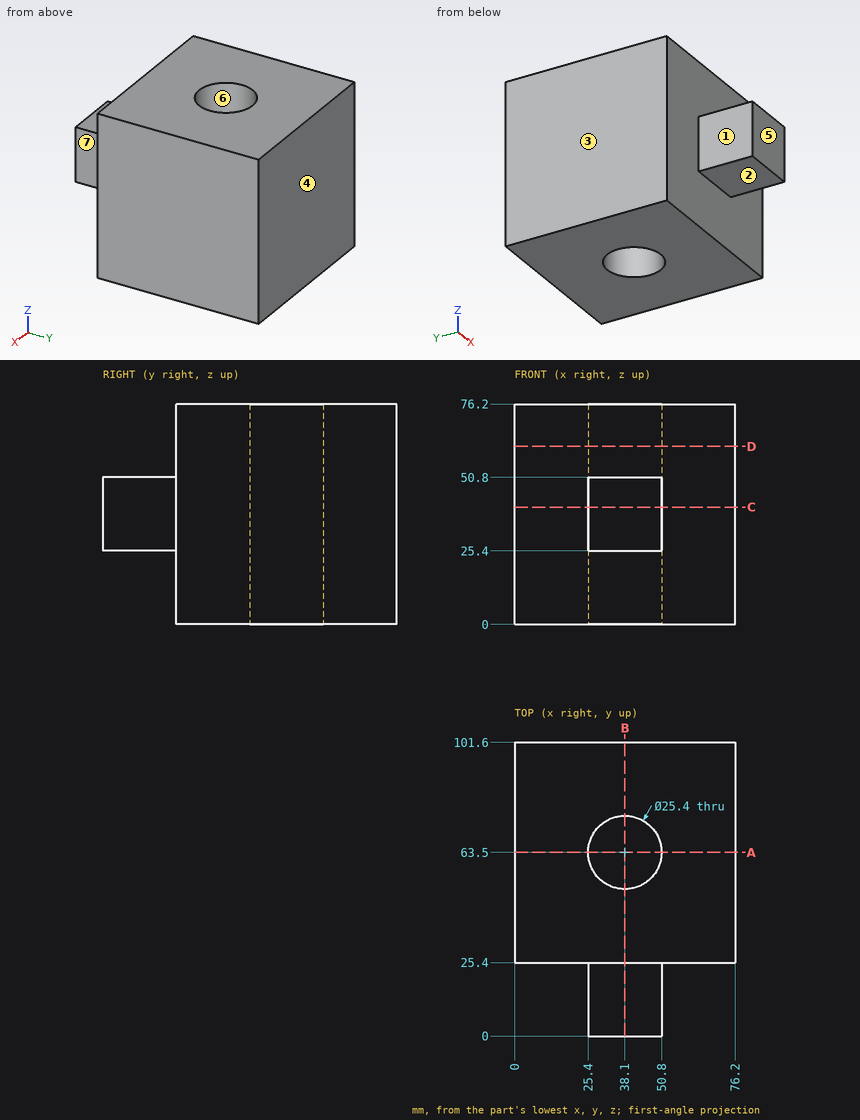
Part print with two shaded views. Sizes in mm from the minimum x, y, z corner. A direction names the side the tool comes from. Round coordinates to 2 decimals unless told otherwise and drop trailing zeros. Loops run counter-clockwise (first coordinate to the right, second up) from the corner with the lowest first, then second, coordinate; pieces in that order, holes last. Notation, with made-up numbers: M 45.5,79 L 89.5,79 A19 cw 89.5,86 Z; hole C 26,-10.5 d10. An arc over 180 degrees is marked long. Put each result on its own line as item: value. Start each with the question number.
Item 1: Drop flat-ended pins along their axis: P1, Ø12.5, axis at y = 14.5, z = 39.5, coming from the +X side; P2, Ø20.5, axis at x = 38.1, y = 63.5, coming from the +Z side; P3, Ø8, axis at y = 57, z = 40, coming from the -X side; P4, Ø12.5, axis at x = 41.5, y = 16.5, coming from the +Z side. Give the stop position or say it passes through.
Item 2: Cut at C-C (z = 40.5). List the corners of the cut face in (x, y), then the cut area to 3 significant figures.
Item 3: Cut at D-D (z = 61.5). List the corners of the cut face in (x, y), then the cut area to 3 significant figures.
Item 4: 3-axis set-ups, long thin cutter, end or side, ignore diameter. For the marked faces 1, 2 and 3: which of +Z, -Z, +X, -X, +Y, -Y reach the whole face in a straight line?
Item 5: Drill centre lines: line 1 along Y through (x, z) = (38, 20); line 2 along Y through (x, z) = (38.1, 29); line 3 along Z through (x, y) = (35, 25). Where is each one in solid material? Low to high.
Item 6: Cut at A-A (y = 63.5). List the corners of the cut face in (x, z).
Item 7: Cut at B-B (x = 38.1). List the corners of the cut face in (y, z), then the cut area to 3 significant figures.
Item 8: Mould opens along Y. For the marked faces 4, 5, 6 and 7 say: released by +Y, released by -Y, zero draft, split by the parting line, or undercut.
Answer block:
1. P1: x = 50.8
1. P2: through
1. P3: x = 0
1. P4: z = 50.8
2. outline: M 0,25.4 L 25.4,25.4 L 25.4,0 L 50.8,0 L 50.8,25.4 L 76.2,25.4 L 76.2,101.6 L 0,101.6 Z; hole C 38.1,63.5 d25.4
2. area: 5,940 mm2
3. outline: M 0,25.4 L 76.2,25.4 L 76.2,101.6 L 0,101.6 Z; hole C 38.1,63.5 d25.4
3. area: 5,300 mm2
4. face 1: +Z, -Z, -X, -Y
4. face 2: -Z, +X, -X, -Y
4. face 3: +Z, -Z, -X, +Y, -Y
5. line 1: 25.4 to 50.8, 76.2 to 101.6
5. line 2: 0 to 50.8, 76.2 to 101.6
5. line 3: 25.4 to 50.8
6. outline: M 0,0 L 25.4,0 L 25.4,76.2 L 0,76.2 Z; M 50.8,0 L 76.2,0 L 76.2,76.2 L 50.8,76.2 Z
7. outline: M 0,25.4 L 25.4,25.4 L 25.4,0 L 50.8,0 L 50.8,76.2 L 25.4,76.2 L 25.4,50.8 L 0,50.8 Z; M 76.2,0 L 101.6,0 L 101.6,76.2 L 76.2,76.2 Z
7. area: 4,520 mm2
8. face 4: released by +Y
8. face 5: released by -Y
8. face 6: undercut
8. face 7: zero draft
